from build123d import *

# Parameters (mm, degrees)
CUT_EXTRUDE1_DEPTH      = 63.353829072
CUT_EXTRUDE1_DEPTH_BACK = 63.353829072
CUT_EXTRUDE2_DEPTH      = 62.546730387
CUT_EXTRUDE2_DEPTH_BACK = 62.546730387


with BuildPart() as part:
    # Sketch1 → Revolve1 (revolve)
    with BuildSketch(Plane.XY, mode=Mode.PRIVATE) as revolve1_sk:
        Polygon((12, 0), (26, 0), (36, 36), (28, 36), (20.5, 9), (12, 9), align=None)
    revolve(revolve1_sk.sketch.rotate(Axis((0, 54.736842105, 0), (0, -1, 0)), 90), axis=Axis((0, 54.736842105, 0), (0, -1, 0)))

    # Sketch2 → Cut-Extrude1 (cut, two sides: drawn at the far end of the back side and taken through both)
    with BuildSketch(Plane(origin=(0, 0, 0), x_dir=(0, 0, -1), z_dir=(1, 0, 0)).offset(-CUT_EXTRUDE1_DEPTH_BACK)):
        with BuildLine():
            Line((-10, 36), (10, 36))
            ThreePointArc((10, 36), (0, 26), (-10, 36))
        make_face()
    extrude(amount=CUT_EXTRUDE1_DEPTH + CUT_EXTRUDE1_DEPTH_BACK, mode=Mode.SUBTRACT)

    # Sketch3 → Cut-Extrude2 (cut, two sides: drawn at the far end of the back side and taken through both)
    with BuildSketch(Plane.XY.offset(-CUT_EXTRUDE2_DEPTH_BACK)):
        with BuildLine():
            Line((-10, 36), (10, 36))
            ThreePointArc((10, 36), (0, 26), (-10, 36))
        make_face()
    extrude(amount=CUT_EXTRUDE2_DEPTH + CUT_EXTRUDE2_DEPTH_BACK, mode=Mode.SUBTRACT)


solid = part.part
Input: part model. Units: mm. Frame: model coordinates. A direction names the side the tool comes from. Give positions to 0.01 mm unless a question says otherwise; leave off trailing zeros. Loops run counter-clockwise (first coordinate to the right, second up) from the corner with the lowest first, then second, coordinate; pieces in that order, holes last. Notation, with made-up numbers: M -11.5,25 L 5.5,25 A34 ccw 5.5,62 Z; hole C 85.5,81.25 d9. An arc over 180 degrees is marked long. Use CSV: the item, a comma, the result in double quotes.
(1) Section B-B, the plane x = 0. Return loops of the section in (y, z).
Outcome:
outline,"M 0,-26 L 26,-33.22 L 26,-25.22 L 9,-20.5 L 9,-12 L 0,-12 Z; M 0,12 L 9,12 L 9,20.5 L 26,25.22 L 26,33.22 L 0,26 Z"
(2) Material intervals for L1, parallel to Y at x = 8.5, z = -15.5; L2, parallel to X at y = 6, z = 0; L3, parallel to X at y = 11.5, z = -9, sorted ascending. Write a range as [from, to].
Outcome:
L1,"y = [0, 9]"
L2,"x = [-27.67, -12], [12, 27.67]"
L3,"x = [-27.77, -19.19], [19.19, 27.77]"
(3) Section A-A, the plane z = 0. Return loops of the section in (x, y).
Outcome:
outline,"M -33.22,26 L -26,0 L -12,0 L -12,9 L -20.5,9 L -25.22,26 Z; M 12,0 L 26,0 L 33.22,26 L 25.22,26 L 20.5,9 L 12,9 Z"
(4) Set-up query: faces 4 (the face through (0, 26, 30)), 5 (the face through (9, 9, 9)). Return all of +Z, -Z, +X, -X, +Y, -Y with unobstructed straight access to the full face (end or side cutting, diameter ignored); none if empty.
Outcome:
face 4,"+Z, -Z, +Y"
face 5,"+Y"
(5) Section D-D, the plane y = 8. Return loops of the section in (x, z).
Outcome:
outline,"C 0,0 d56.44; hole C 0,0 d24"
(6) Pin query (flat end, axial travel): P1, Ø4, axis at y = 14.5, z = -21, coming from the -X side; P2, Ø2, axis at x = 19.5, y = 24, coming from the +Z side; P3, Ø1.5, axis at y = 6.5, z = 4, coming from the -X side. Return the tip coordinate at first contact, or that it passes through.
Outcome:
P1,"stops at x = -23.4"
P2,"stops at z = 27"
P3,"stops at x = -27.75"
(7) Section C-C, the plane y = 21.5. Return loops of the section in (x, z), plus the area to 3 significant figures.
Outcome:
outline,"C 0,0 d63.94; hole C 0,0 d47.94"
area,"1,410 mm²"
(8) Pull-direction query (Z, two-part tool) for faces 1 (the face through (-3.604, 4.437, 11.446)), 2 (the face through (-8.665, 10.252, 27.516)), 3 (the face through (-22, 36, -22)); classes: pulls with the +Z half, pulls with the -Z half, needs draft (parallel to the pull), parting line crosses it, or undercut.
Outcome:
face 1,"undercut"
face 2,"parting line crosses it"
face 3,"needs draft"
